For this review, take the finished solid that the model builds, in its own axes (mm). A direction names the side the tool comes from. Coordinates: 2 decimals unless noted, no trailing zeros. Write each loop counter-clockwise with the first axis right and the second up, starting at its lowest first coordinate (ties: lowest second). Pieces come first, ordered by that corner, then holes. Notation, with made-up numbers: M -33,58 L 10,58 A27 cw 10,84 Z; hole C 26,62.25 d8. An arc over 180 degrees is marked long. One line per question, with ' | ' between items.
from build123d import *

# Parameters (mm, degrees)
SKETCH_1_R               = 14
EXTRUDE_1_DEPTH          = 6
SKETCH_2_R               = 10
EXTRUDE_2_DEPTH          = 15
SKETCH_3_R               = 1
SKETCH_3_R_2             = 4
CUT_EXTRUDE_1_DEPTH      = 5
CUT_EXTRUDE_2_DEPTH      = 5
PATTERN_CIRCULAR_1_COUNT = 4
SKETCH_5_R               = 4
CUT_EXTRUDE_3_DEPTH      = 22


with BuildPart() as part:
    # Эскиз1 → Бобышка-Вытянуть1 (new body)
    with BuildSketch(Plane(origin=(0, 0, 0), x_dir=(1, 0, 0), z_dir=(0, 1, 0))):
        Circle(SKETCH_1_R)
    extrude(amount=EXTRUDE_1_DEPTH)

    # Эскиз2 → Бобышка-Вытянуть2 (add)
    with BuildSketch(Plane(origin=(0, 6, 0), x_dir=(1, 0, 0), z_dir=(0, 1, 0))):
        Circle(SKETCH_2_R)
    extrude(amount=EXTRUDE_2_DEPTH)

    # Эскиз3 → Вырез-Вытянуть1 (cut)
    with BuildSketch(Plane.XZ):
        with Locations((-8, 0)):
            Circle(SKETCH_3_R)
        with Locations((8, 0)):
            Circle(SKETCH_3_R)
        with Locations((0, 9.5)):
            Circle(SKETCH_3_R)
        with Locations((0, -9.5)):
            Circle(SKETCH_3_R)
        with Locations((-7.778174593, 7.778174593)):
            Circle(SKETCH_3_R_2)
        with Locations((7.778174593, 7.778174593)):
            Circle(SKETCH_3_R_2)
        with Locations((7.778174593, -7.778174593)):
            Circle(SKETCH_3_R_2)
        with Locations((-7.778174593, -7.778174593)):
            Circle(SKETCH_3_R_2)
    extrude(amount=-CUT_EXTRUDE_1_DEPTH, mode=Mode.SUBTRACT)

    # Эскиз4 → Вырез-Вытянуть2 (cut)
    with BuildSketch(Plane.XZ):
        Polygon((-4.949747468, 10.606601718), (-10.606601718, 4.949747468), (-15.333238313, 9.676384064), (-9.676384064, 15.333238313), align=None)
    cut_extrude_2 = extrude(amount=-CUT_EXTRUDE_2_DEPTH, mode=Mode.SUBTRACT)

    # Круговой массив1: Вырез-Вытянуть2 ×4 about axis
    pattern_circular_1_axis = Axis((0, 0, 0), (0, 1, 0))
    for i in range(1, PATTERN_CIRCULAR_1_COUNT):
        add(cut_extrude_2.rotate(pattern_circular_1_axis, i * 360 / PATTERN_CIRCULAR_1_COUNT), mode=Mode.SUBTRACT)

    # Эскиз5 → Вырез-Вытянуть3 (cut, through all)
    with BuildSketch(Plane.XZ):
        Circle(SKETCH_5_R)
    extrude(amount=-CUT_EXTRUDE_3_DEPTH, mode=Mode.SUBTRACT)


solid = part.part
1. Take a section at B-B on y = 2.75. State the section outline as (x, z) points.
Computed values:
outline: M -12.32,-6.66 L -10.61,-4.95 A4 cw -4.95,-10.61 L -6.66,-12.32 A14 ccw 6.66,-12.32 L 4.95,-10.61 A4 cw 10.61,-4.95 L 12.32,-6.66 A14 ccw 12.32,6.66 L 10.61,4.95 A4 cw 4.95,10.61 L 6.66,12.32 A14 ccw -6.66,12.32 L -4.95,10.61 A4 cw -10.61,4.95 L -12.32,6.66 A14 ccw Z; hole C -8,0 d2; hole C 0,0 d8; hole C 0,-9.5 d2; hole C 0,9.5 d2; hole C 8,0 d2
2. Take a section at A-A on z = 0. State the section outline as (x, y) points, plus the area to 3 significant figures.
Computed values:
outline: M -14,0 L -9,0 L -9,5 L -7,5 L -7,0 L -4,0 L -4,21 L -10,21 L -10,6 L -14,6 Z; M 4,0 L 7,0 L 7,5 L 9,5 L 9,0 L 14,0 L 14,6 L 10,6 L 10,21 L 4,21 Z | area: 280 mm2
3. Machinability: for faces 4 (the flat face through (-5.792, 2.465, -11.449)), 5 (the flat face through (11.473, 2.465, 5.816)), 6 (the flat face through (5.816, 2.465, -11.473)), 7 (the cylindrical face through (4.9, 2.5, 5)), which of the approach directions +Z, -Z, +X, -X, +Y, -Y give a long, thin tool a straight path to every point of the face, cutting with its end or side? Answer none if there is none.
Computed values:
face 4: -X, -Y | face 5: +Z, -Y | face 6: +X, -Y | face 7: -Y
4. Take a section at D-D on y = 15.5. State the section outline as (x, z) points, plus the area to 3 significant figures.
Computed values:
outline: C 0,0 d20; hole C 0,0 d8 | area: 264 mm2
5. Clearance check with flat-ended pins moving along their axes: P1, Ø2.5, axis at x = -9.5, z = -6.5, coming from the -Y side; P2, Ø3, axis at x = -5, y = 11, coming from the +Z side; P3, Ø1.5, axis at y = 17, z = 2, coming from the -X side. State where each tip first meets the part, or that it passes through.
Computed values:
P1: stops at y = 5 | P2: stops at z = 9.37 | P3: stops at x = -9.92
6. Take a section at C-C on x = 0. State the section outline as (y, z) points.
Computed values:
outline: M 0,-14 L 6,-14 L 6,-10 L 21,-10 L 21,-4 L 0,-4 L 0,-8.5 L 5,-8.5 L 5,-10.5 L 0,-10.5 Z; M 0,4 L 21,4 L 21,10 L 6,10 L 6,14 L 0,14 L 0,10.5 L 5,10.5 L 5,8.5 L 0,8.5 Z
7. Draft analysis for pull direction Z (two halves, no side actions). For faces 1 (the cylindrical face through (-2.17, 13.4, 9.76)), 2 (the flat face through (8, 5, -7)), 3 (the flat face through (-3, 6, -10)), state which applies: pulls with the +Z half, pulls with the -Z half, needs draft (parallel to the pull), parting line crosses it, or undercut.
Computed values:
face 1: parting line crosses it | face 2: undercut | face 3: needs draft
8. For line 1 along Z through (x, y) = (8, 1.05); line 2 along X through (y, z) = (10.25, 0.25); line 3 along Z through (x, y) = (0, 1.65), list the stretches that pass through material, from the lowest coordinate up.
Computed values:
line 1: z = -3.78 to -1, 1 to 3.78 | line 2: x = -10 to -3.99, 3.99 to 10 | line 3: z = -14 to -10.5, -8.5 to -4, 4 to 8.5, 10.5 to 14
